from build123d import *

# Parameters (mm, degrees)
F0_R      = 3.575
F1_DEPTH  = 2.1
F2_R      = 1.6
F3_DEPTH  = 8.25
F4_R      = 4.44
F4_R_2    = 1.6
F5_DEPTH  = 2.6
F6_R      = 1.0460304523
F7_R      = 2.3939824527
F8_R      = 2.025
F10_R     = 0.575
F11_DEPTH = 8.2
F12_R     = 0.2
F13_DEPTH = 3.2
F14_R     = 0.575
F15_R     = 0.2


with BuildPart() as f1:
    # F0 (on Top) → F1 (new body)
    with BuildSketch(Plane.XY):
        Circle(F0_R)
    extrude(amount=F1_DEPTH)

    # F2 (on face) → F3 (join)
    with BuildSketch(Plane.XY.offset(2.1)):
        Circle(F2_R)
    extrude(amount=F3_DEPTH)

    # F4 (on face) → F5 (join)
    with BuildSketch(Plane.XY.offset(10.35)):
        Circle(F4_R)
        Circle(F4_R_2, mode=Mode.SUBTRACT)
    extrude(amount=-F5_DEPTH)

    # F6
    f6_edges = [f1.edges().sort_by_distance(p)[0] for p in [
        (-3.575, 0, 2.1),
        (-3.575, 0, 0),
    ]]
    fillet(f6_edges, radius=F6_R)

    # F7
    f7_edges = [f1.edges().sort_by_distance(p)[0] for p in [
        (-4.44, 0, 7.75),
    ]]
    fillet(f7_edges, radius=F7_R)

    # F2 (on face) → F9 section 0
    with BuildSketch(Plane.XY.offset(2.1)):
        Circle(F2_R)
    # F8 (on face) → F9 section 1
    with BuildSketch(Plane(origin=(0, 0, 7.75), x_dir=(1, 0, 0), z_dir=(0, 0, -1))):
        Circle(F8_R)
    loft()

    # F10 (on face) → F11 (join)
    with BuildSketch(Plane.XY.offset(10.35)):
        Circle(F10_R)
    extrude(amount=F11_DEPTH)

    # F12 (on face) → F13 (join)
    with BuildSketch(Plane.XY.offset(18.55)):
        Circle(F12_R)
    extrude(amount=F13_DEPTH)

    # F14 (on face) → F16 section 0
    with BuildSketch(Plane.XY.offset(18.55)):
        Circle(F14_R)
    # F15 (on face) → F16 section 1
    with BuildSketch(Plane.XY.offset(21.75)):
        Circle(F15_R)
    loft()


solid = f1.part
Build history of the part. All positions in model axes, mm. Round coordinates to 2 decimals unless told otherwise and drop trailing zeros. Write each loop counter-clockwise with the first axis right and the second up, starting at its lowest first coordinate (ties: lowest second). Pieces come first, ordered by that corner, then holes. Notation, with made-up numbers: M -25.5,11 L -7.5,11 A18 cw -7.5,24 Z; hole C 56,23 d2. An arc over 180 degrees is marked long. Answer as a JSON object with one key per item and string values. Group by question number.
(1) Mould opens along Z. For faces 1 (the conical face through (-1.441, -1.105, 4.965)), 2 (the flat face through (0, 0, 0)), 3 (the conical face through (-0.083, -0.376, 20.172)), 4 (the flat face through (0, -2, 2.1)) say: pulls with the +Z half, pulls with the -Z half, needs draft (parallel to the pull), parting line crosses it, or undercut.
(2) Flat gauge pins, fed straight in: pin 1 (4 mm diameter, centred on y = 3, z = 16.5, fed in from +X); pin 2 (1 mm diameter, centred on x = -0.5, z = 8.5, fed in from -Y); pin 3 (1.5 mm diameter, centred on x = 2, y = -0.5, fed in from +Z); pin 4 (3 mm diameter, centred on x = -1.5, z = 19, fed in from -Y). Where does each tip first touch, or does it go through?
(3) Cut at A-A (z = 18). Give the cut face in (x, y) (3 decimals), and give its area (3 significant figures).
(4) Cut at B-B (z = 3.75). Give the cut face in (x, y).
(5) Drill centre lines: L1, parallel to Z at x = 2, y = -0.75; L2, parallel to Z at x = 2.75, y = 0; L3, parallel to Z at x = 2.75, y = 2.5. Where is each one in solid material? Low to high.
Responses:
{
 "1": {"face 1": "undercut", "face 2": "pulls with the -Z half", "face 3": "pulls with the +Z half", "face 4": "undercut"},
 "2": {"pin 1": "passes through", "pin 2": "stops at y = -4.12", "pin 3": "stops at z = 10.35", "pin 4": "stops at y = -0.57"},
 "3": {"outline": "C 0,0 d1.15", "area": "1.04 mm2"},
 "4": {"outline": "C 0,0 d3.45"},
 "5": {"L1": "z = 0 to 2.1, 7.75 to 10.35", "L2": "z = 0.02 to 2.08, 7.86 to 10.35", "L3": "z = 8.43 to 10.35"}
}
